```python
from build123d import *

# Parameters (mm, degrees)
ESQUISSE1_W             = 180
ESQUISSE1_H             = 250
BOSS_EXTRU_1_DEPTH      = 15
ESQUISSE2_R             = 2.25
ENL_V_MAT_EXTRU_1_DEPTH = 15
ESQUISSE3_R             = 2.25
ENL_V_MAT_EXTRU_2_DEPTH = 15
ESQUISSE6_W             = 40
ESQUISSE6_H             = 52
ENL_V_MAT_EXTRU_4_DEPTH = 3
ESQUISSE4_W             = 39
ESQUISSE4_H             = 40
ESQUISSE4_W_2           = 12
ENL_V_MAT_EXTRU_3_DEPTH = 3
ENL_V_START             = -15
ESQUISSE7_R             = 2.5
ENL_V_MAT_EXTRU_5_DEPTH = 15
ESQUISSE8_W             = 52
ESQUISSE8_H             = 40
ENL_V_MAT_EXTRU_6_DEPTH = 3
ESQUISSE9_W             = 40
ESQUISSE9_H             = 12
ENL_V_MAT_EXTRU_7_DEPTH = 3
ESQUISSE10_W            = 40
ESQUISSE10_H            = 60
ENL_V_MAT_EXTRU_8_DEPTH = 3
ESQUISSE11_W            = 58.5
ESQUISSE11_H            = 40
ENL_V_MAT_EXTRU_9_DEPTH = 3


with BuildPart() as part:
    # Esquisse1 → Boss.-Extru.1 (new body)
    with BuildSketch(Plane.XY):
        with Locations((90, 125)):
            Rectangle(ESQUISSE1_W, ESQUISSE1_H)
    extrude(amount=BOSS_EXTRU_1_DEPTH)

    # Esquisse2 → Enlèv. mat.-Extru.1 (cut)
    with BuildSketch(Plane.XY.offset(15)):
        with Locations((11.5, 184.5)):
            Circle(ESQUISSE2_R)
        with Locations((37.5, 184.5)):
            Circle(ESQUISSE2_R)
        with Locations((37.5, 156.5)):
            Circle(ESQUISSE2_R)
        with Locations((11.5, 156.5)):
            Circle(ESQUISSE2_R)
        with Locations(Location((168.5, 156.5, 0), (0, 0, 180))):
            Circle(ESQUISSE2_R)
        with Locations(Location((142.5, 156.5, 0), (0, 0, 180))):
            Circle(ESQUISSE2_R)
        with Locations(Location((142.5, 184.5, 0), (0, 0, 180))):
            Circle(ESQUISSE2_R)
        with Locations(Location((168.5, 184.5, 0), (0, 0, 180))):
            Circle(ESQUISSE2_R)
        with Locations((168.5, 15.5)):
            Circle(ESQUISSE2_R)
        with Locations((142.5, 15.5)):
            Circle(ESQUISSE2_R)
        with Locations((142.5, 43.5)):
            Circle(ESQUISSE2_R)
        with Locations((168.5, 43.5)):
            Circle(ESQUISSE2_R)
        with Locations(Location((11.5, 43.5, 0), (0, 0, 180))):
            Circle(ESQUISSE2_R)
        with Locations(Location((37.5, 43.5, 0), (0, 0, 180))):
            Circle(ESQUISSE2_R)
        with Locations(Location((37.5, 15.5, 0), (0, 0, 180))):
            Circle(ESQUISSE2_R)
        with Locations(Location((11.5, 15.5, 0), (0, 0, 180))):
            Circle(ESQUISSE2_R)
        with Locations((78, 120)):
            Circle(ESQUISSE2_R)
        with Locations(Location((78, 80, 0), (0, 0, 180))):
            Circle(ESQUISSE2_R)
        with Locations((102, 80)):
            Circle(ESQUISSE2_R)
        with Locations(Location((102, 120, 0), (0, 0, 180))):
            Circle(ESQUISSE2_R)
    extrude(amount=-ENL_V_MAT_EXTRU_1_DEPTH, mode=Mode.SUBTRACT)

    # Esquisse3 → Enlèv. mat.-Extru.2 (cut)
    with BuildSketch(Plane.XY.offset(15)):
        with Locations((12, 226)):
            Circle(ESQUISSE3_R)
        with Locations((40, 226)):
            Circle(ESQUISSE3_R)
        with Locations((12, 200)):
            Circle(ESQUISSE3_R)
        with Locations((40, 200)):
            Circle(ESQUISSE3_R)
        with Locations(Location((140, 200, 0), (0, 0, 180))):
            Circle(ESQUISSE3_R)
        with Locations(Location((168, 200, 0), (0, 0, 180))):
            Circle(ESQUISSE3_R)
        with Locations(Location((140, 226, 0), (0, 0, 180))):
            Circle(ESQUISSE3_R)
        with Locations(Location((168, 226, 0), (0, 0, 180))):
            Circle(ESQUISSE3_R)
        with Locations((168, 74)):
            Circle(ESQUISSE3_R)
        with Locations((140, 74)):
            Circle(ESQUISSE3_R)
        with Locations((168, 100)):
            Circle(ESQUISSE3_R)
        with Locations((140, 100)):
            Circle(ESQUISSE3_R)
        with Locations(Location((40, 100, 0), (0, 0, 180))):
            Circle(ESQUISSE3_R)
        with Locations(Location((12, 100, 0), (0, 0, 180))):
            Circle(ESQUISSE3_R)
        with Locations(Location((40, 74, 0), (0, 0, 180))):
            Circle(ESQUISSE3_R)
        with Locations(Location((12, 74, 0), (0, 0, 180))):
            Circle(ESQUISSE3_R)
    extrude(amount=-ENL_V_MAT_EXTRU_2_DEPTH, mode=Mode.SUBTRACT)

    # Esquisse6 → Enlèv. mat.-Extru.4 (cut)
    with BuildSketch(Plane(origin=(0, 0, 0), x_dir=(-1, 0, 0), z_dir=(0, 0, -1))):
        with Locations((-90, 100)):
            Rectangle(ESQUISSE6_W, ESQUISSE6_H)
    extrude(amount=-ENL_V_MAT_EXTRU_4_DEPTH, mode=Mode.SUBTRACT)

    # Esquisse4 → Enlèv. mat.-Extru.3 (cut)
    with BuildSketch(Plane(origin=(0, 0, 0), x_dir=(-1, 0, 0), z_dir=(0, 0, -1))):
        with Locations((-155.5, 170.5)):
            Rectangle(ESQUISSE4_W, ESQUISSE4_H)
        with Locations((-155.5, 29.5)):
            Rectangle(ESQUISSE4_W, ESQUISSE4_H)
        with Locations((-24.5, 29.5)):
            Rectangle(ESQUISSE4_W, ESQUISSE4_H)
        with Locations((-24.5, 170.5)):
            Rectangle(ESQUISSE4_W, ESQUISSE4_H)
        with Locations((-115.5, 100)):
            Rectangle(ESQUISSE4_W_2, ESQUISSE4_H)
        with Locations((-64.5, 100)):
            Rectangle(ESQUISSE4_W_2, ESQUISSE4_H)
    extrude(amount=-ENL_V_MAT_EXTRU_3_DEPTH, mode=Mode.SUBTRACT)

    # Esquisse7 → Enlèv. mat.-Extru.5 (cut)
    with BuildSketch(Plane.XY.offset(15).offset(ENL_V_START)):
        with Locations((70, 172)):
            Circle(ESQUISSE7_R)
        with Locations(Location((110, 172, 0), (0, 0, 180))):
            Circle(ESQUISSE7_R)
        with Locations((110, 148)):
            Circle(ESQUISSE7_R)
        with Locations(Location((70, 148, 0), (0, 0, 180))):
            Circle(ESQUISSE7_R)
    extrude(amount=ENL_V_MAT_EXTRU_5_DEPTH, mode=Mode.SUBTRACT)

    # Esquisse8 → Enlèv. mat.-Extru.6 (cut)
    with BuildSketch(Plane.XY.offset(15)):
        with Locations((90, 160)):
            Rectangle(ESQUISSE8_W, ESQUISSE8_H)
    extrude(amount=-ENL_V_MAT_EXTRU_6_DEPTH, mode=Mode.SUBTRACT)

    # Esquisse9 → Enlèv. mat.-Extru.7 (cut)
    with BuildSketch(Plane.XY.offset(15)):
        with Locations((90, 134)):
            Rectangle(ESQUISSE9_W, ESQUISSE9_H)
        with Locations((90, 186)):
            Rectangle(ESQUISSE9_W, ESQUISSE9_H)
    extrude(amount=-ENL_V_MAT_EXTRU_7_DEPTH, mode=Mode.SUBTRACT)

    # Esquisse10 → Enlèv. mat.-Extru.8 (cut)
    with BuildSketch(Plane.XY.offset(15)):
        with Locations((90, 220)):
            Rectangle(ESQUISSE10_W, ESQUISSE10_H)
    extrude(amount=-ENL_V_MAT_EXTRU_8_DEPTH, mode=Mode.SUBTRACT)

    # Esquisse11 → Enlèv. mat.-Extru.9 (cut)
    with BuildSketch(Plane(origin=(0, 0, 0), x_dir=(-1, 0, 0), z_dir=(0, 0, -1))):
        with Locations((-29.25, 100)):
            Rectangle(ESQUISSE11_W, ESQUISSE11_H)
        with Locations((-150.75, 100)):
            Rectangle(ESQUISSE11_W, ESQUISSE11_H)
    extrude(amount=-ENL_V_MAT_EXTRU_9_DEPTH, mode=Mode.SUBTRACT)


solid = part.part
```
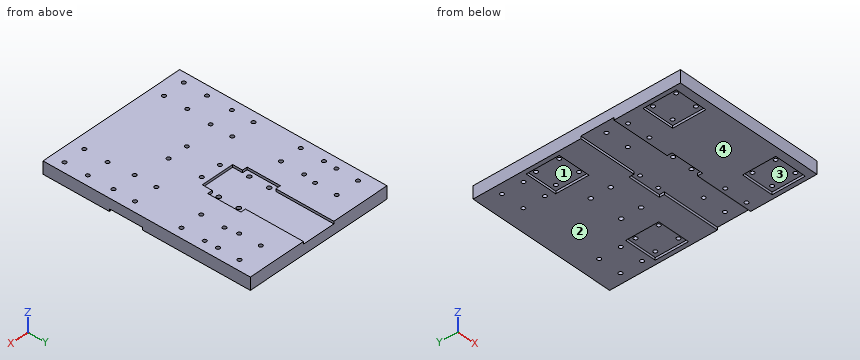
Could you check a few things on this model? Use its own coordinates, in mm. Face numbers are marked on the shaded views. A direction names the side the tool comes from. Round coordinates to 2 decimals unless told otherwise and drop trailing zeros. Write each loop counter-clockwise with the first axis right and the second up, starting at its lowest first coordinate (ties: lowest second). Pieces come first, ordered by that corner, then holes. Notation, with made-up numbers: M 12,89 L 46,89 A5 cw 46,93 Z; hole C 5,35 d6. An arc over 180 degrees is marked long. Write each question's results on one line, items separated by ' | '. Start each with the question number.
1. I need wall thicknesses on L1, parallel to Y at x = 140, z = 4.75; L2, parallel to Y at x = 171.5, z = 2.25; L3, parallel to X at y = 148, z = 7.5. Which ranges of each line are inside material? Lowest first, please. Write a range as from..to.
2. Imagine slicing it at A-A on y = 148. List the corners of the cut face in (x, z) for me, and give its area (3 significant figures).
3. Imagine slicing it at D-D on y = 93.5. List the corners of the cut face in (x, z) for me.
4. Thinking about a two-plate mould opening in X: for the marked faces 1 and 2, which applies, +X half, -X half, draft (parallel to the pull), parting line (faces both ways), or undercut?
5. Imagine slicing it at C-C on x = 29. List the corners of the cut face in (y, z) for me.
6. Imagine slicing it at B-B on y = 31.5. List the corners of the cut face in (x, z) for me.
7. I'm going to push flat-ended pins straight in: pin 1 Ø4 at (x, y) = (11.5, 184.5) entering from +Z; pin 2 Ø5 at (x, y) = (142.5, 15.5) entering from -Z. Where does each tip first touch, or does it pass through?
8. On a 3-axis mill with a long thin cutter (end or side, diameter ignored), from which of +Z, -Z, +X, -X, +Y, -Y can I reach the whole of each face in a straight line? I mean the marked faces 3 and 4. Say none if no direction works.
Result sheet:
1) L1: y = 0..71.75, 76.25..97.75, 102.25..197.75, 202.25..223.75, 228.25..250 | L2: y = 0..9.5, 49.5..80, 120..150.5, 190.5..250 | L3: x = 0..67.5, 72.5..107.5, 112.5..180
2) outline: M 0,0 L 67.5,0 L 67.5,12 L 64,12 L 64,15 L 0,15 Z; M 72.5,0 L 107.5,0 L 107.5,12 L 72.5,12 Z; M 112.5,0 L 180,0 L 180,15 L 116,15 L 116,12 L 112.5,12 Z | area: 2,420 mm^2
3) outline: M 0,3 L 180,3 L 180,15 L 0,15 Z
4) face 1: undercut | face 2: draft
5) outline: M 0,0 L 9.5,0 L 9.5,3 L 49.5,3 L 49.5,0 L 80,0 L 80,3 L 120,3 L 120,0 L 150.5,0 L 150.5,3 L 190.5,3 L 190.5,0 L 250,0 L 250,15 L 0,15 Z
6) outline: M 0,0 L 5,0 L 5,3 L 44,3 L 44,0 L 136,0 L 136,3 L 175,3 L 175,0 L 180,0 L 180,15 L 0,15 Z
7) pin 1: passes through | pin 2: stops at z = 3
8) face 3: -Z | face 4: -Z, +X, -X, +Y, -Y
